Work out the finished part from the listing and answer in its coordinate system (mm). Face numbers are marked on the shaded views. A direction names the side the tool comes from. Give positions to 0.01 mm unless a question says otherwise; leave off trailing zeros. Order: outer loops, then holes, each group sorted by start corner. A loop starts at its lowest first (then second) coordinate and runs counter-clockwise, first axis right, second up. Notation, with made-up numbers: (70.5, 9) - (85.5, 9) arc R9 cw to (85.5, 21) - close; hole circle Ø2 at (41, 2.5). An arc over 180 degrees is marked (long way). Write each question's results on one line, items separated by ' | '.
from build123d import *

# Parameters (mm, degrees)
RESSALTO_EXTRUS_O1_DEPTH  = 15
ESBO_O7_W                 = 30
ESBO_O7_H                 = 15
RESSALTO_EXTRUS_O3_DEPTH  = 3
ESBO_O14_W                = 7
ESBO_O14_H                = 107.753429602
RESSALTO_EXTRUS_O5_DEPTH  = 2
ESBO_O15_W                = 7
ESBO_O15_H                = 107.852923352
RESSALTO_EXTRUS_O6_DEPTH  = 2
ESBO_O16_W                = 7
ESBO_O16_H                = 22.5
RESSALTO_EXTRUS_O9_DEPTH  = 2
CHANFRO11_SIZE            = 20.026147127
CHANFRO11_SIZE_2          = 10
CHANFRO12_SIZE            = 5.181688732
CHANFRO12_SIZE_2          = 10
CHANFRO13_SIZE            = 2
CHANFRO14_SIZE            = 4.8
CHANFRO14_SIZE2           = 5.970145796
CHANFRO16_SIZE            = 1.5
CHANFRO17_SIZE            = 1.5
CHANFRO18_SIZE            = 1
ESBO_O17_R                = 2
CORTE_EXTRUS_O1_DEPTH     = 5
CHANFRO20_SIZE            = 1
RESSALTO_EXTRUS_O10_DEPTH = 7
RESSALTO_EXTRUS_O11_DEPTH = 2
RESSALTO_EXTRUS_O13_DEPTH = 2
ESBO_O23_W                = 5
ESBO_O23_H                = 10
CORTE_EXTRUS_O2_DEPTH     = 60
CHANFRO22_SIZE            = 1.5
CHANFRO21_SIZE            = 1


# Some blends are built 0.0001 mm under size
with BuildPart() as part:
    # Esboço2 → Ressalto-extrusão1 (new body)
    with BuildSketch(Plane.XY):
        Polygon((-41.65, 8.85), (-41.65, 11.85), (-50.65, 11.85), (-50.65, -10.65), (-27.65, -10.65), (-27.65, -7.65), (-47.65, -7.65), (-47.65, 8.85), align=None)
    extrude(amount=RESSALTO_EXTRUS_O1_DEPTH)



with BuildPart() as body_2:
    # Esboço7 → Ressalto-extrusão3 (new body)
    with BuildSketch(Plane(origin=(0, -117.65, 0), x_dir=(-1, 0, 0), z_dir=(0, -1, 0))):
        with Locations((59.65, -7.5)):
            Rectangle(ESBO_O7_W, ESBO_O7_H)
    extrude(amount=-RESSALTO_EXTRUS_O3_DEPTH)


with BuildPart() as part_1:
    add(part.part)

    add(body_2.part)  # Loft3 merges body 2
    # Esboço9 → Loft3 section 0
    with BuildSketch(Plane(origin=(0, -114.65, 0), x_dir=(1, 0, 0), z_dir=(0, 1, 0))):
        with BuildLine():
            Line((-69.65, -15), (-64.65, -15))
            Line((-64.65, -15), (-64.65, 0))
            Line((-64.65, 0), (-69.65, 0))
            Line((-69.65, 0), (-69.65, -15))
        make_face()
    # Esboço8 → Loft3 section 1
    with BuildSketch(Plane.XZ.offset(10.65)):
        with BuildLine():
            Line((-50.65, 15), (-45.65, 15))
            Line((-45.65, 15), (-45.65, 0))
            Line((-45.65, 0), (-50.65, 0))
            Line((-50.65, 0), (-50.65, 15))
        make_face()
    loft()

    # Esboço14 → Ressalto-extrusão5 (add)
    with BuildSketch(Plane(origin=(-42.292744028, 7.726559005, 0), x_dir=(0, 0, -1), z_dir=(0.9837182167305484, -0.17971775113346497, 0))):
        with Locations((-7.5, -70.525331358)):
            Rectangle(ESBO_O14_W, ESBO_O14_H)
    extrude(amount=RESSALTO_EXTRUS_O5_DEPTH)

    # Esboço15 → Ressalto-extrusão6 (add)
    with BuildSketch(Plane(origin=(-47.131251678, 8.610517133, 0), x_dir=(0, 0, 1), z_dir=(-0.9837182167305483, 0.17971775113346522, 0))):
        with Locations((7.5, -73.505764779)):
            Rectangle(ESBO_O15_W, ESBO_O15_H)
    extrude(amount=RESSALTO_EXTRUS_O6_DEPTH)

    # Esboço16 → Ressalto-extrusão9 (add)
    with BuildSketch(Plane.ZY.offset(50.65)):
        with Locations((7.5, 0.6)):
            Rectangle(ESBO_O16_W, ESBO_O16_H)
    extrude(amount=RESSALTO_EXTRUS_O9_DEPTH)

    # Chanfro11
    # the kernel refuses this chamfer: 20.026147127, 10 mm, written as the material it adds along each edge
    with BuildSketch(Plane(origin=(-64.65, -114.65, 55.83646579), x_dir=(0.9998316750706326, -0.018347248443652868, 0), z_dir=(0, 0, -1))) as chanfro11_piece_1_section:
        Polygon((CHANFRO11_SIZE * 0.999831675085, -CHANFRO11_SIZE * 0.0183472484439), (CHANFRO11_SIZE_2 * 0.161638977635, -CHANFRO11_SIZE_2 * 0.986849958661), (0, 0), align=None)
    chanfro11_piece_1 = extrude(amount=55.83646579, mode=Mode.PRIVATE)
    chanfro11_piece_1 = split(chanfro11_piece_1, bisect_by=Plane(origin=(-44.65, -111.70383057, 13), z_dir=(-1, 0, 0)), keep=Keep.TOP, mode=Mode.PRIVATE)
    chanfro11_piece_1 = split(chanfro11_piece_1, bisect_by=Plane(origin=(-56.081001228, -111.70383057, 15), z_dir=(0, 0, -1)), keep=Keep.TOP, mode=Mode.PRIVATE)
    add(chanfro11_piece_1)

    # Chanfro12
    # the kernel refuses this chamfer: 10, 5.181688732 mm, written as the material it adds along each edge
    with BuildSketch(Plane(origin=(-69.65, -114.65, -14.909754714), x_dir=(-0.9981888061534079, -0.06015901653147684, 0), z_dir=(0, 0, 1))) as chanfro12_piece_1_section:
        Polygon((CHANFRO12_SIZE * 0.99818880622, -CHANFRO12_SIZE * 0.0601590165355), (-CHANFRO12_SIZE_2 * 0.238571767911, -CHANFRO12_SIZE_2 * 0.971124869188), (0, 0), align=None)
    chanfro12_piece_1 = extrude(amount=29.909754714, mode=Mode.PRIVATE)
    chanfro12_piece_1 = split(chanfro12_piece_1, bisect_by=Plane(origin=(-74.65, -111.318186465, 5.5), z_dir=(1, 0, 0)), keep=Keep.TOP, mode=Mode.PRIVATE)
    chanfro12_piece_1 = split(chanfro12_piece_1, bisect_by=Plane(origin=(-70.664221075, -111.318186465, 0), z_dir=(0, 0, 1)), keep=Keep.TOP, mode=Mode.PRIVATE)
    add(chanfro12_piece_1)

    # Chanfro13
    chanfro13_edges = [part_1.edges().sort_by_distance(p)[0] for p in [
        (-46.15, 11.85, 15),
        (-46.15, 11.85, 0),
    ]]
    chamfer(chanfro13_edges, length=CHANFRO13_SIZE)

    # Chanfro14
    chanfro14_edges = [part_1.edges().sort_by_distance(p)[0] for p in [
        (-43.616897465, -10.65, 7.5),
    ]]
    chanfro14_side = [part_1.faces().sort_by_distance(p)[0] for p in [
        (-52.309535597, -58.230756092, 7.5),
    ]]
    chamfer(chanfro14_edges, length=CHANFRO14_SIZE, length2=CHANFRO14_SIZE2, reference=chanfro14_side[0])

    # Chanfro16
    chanfro16_edges = [part_1.edges().sort_by_distance(p)[0] for p in [
        (-50.65, 11.85, 3),
        (-51.65, 11.85, 11),
        (-51.65, 11.85, 4),
        (-52.65, 11.85, 7.5),
        (-54.251411244, -57.731408916, 0),
        (-54.251411244, -57.731408916, 15),
        (-53.751411244, -109.724353826, 0),
        (-53.751411244, -109.724353826, 15),
        (-59.251411244, -57.731408916, 15),
        (-59.251411244, -57.731408916, 0),
        (-71.251411244, -109.603357662, 15),
        (-71.251411244, -109.603357662, 0),
        (-50.65, 11.85, 12),
        (-50.65, -0.4, 0),
        (-50.65, 10.85, 1),
        (-50.65, -0.4, 15),
        (-50.65, 10.85, 14),
        (-74.65, -116.021948745, 0),
        (-74.65, -116.021948745, 15),
        (-44.65, -116.14294491, 15),
        (-44.65, -116.14294491, 0),
    ]]
    chamfer(chanfro16_edges, length=CHANFRO16_SIZE)

    # Chanfro17
    chanfro17_edges = [part_1.edges().sort_by_distance(p)[0] for p in [
        (-37.412413451, -10.65, 0),
        (-37.412413451, -10.65, 15),
    ]]
    chamfer(chanfro17_edges, length=CHANFRO17_SIZE)

    # Chanfro18
    chanfro18_edges = [part_1.edges().sort_by_distance(p)[0] for p in [
        (-61.620535422, -59.570685278, 4),
        (-52.65, -0.059403589, 11),
        (-52.7408582, -60.591679812, 4),
        (-61.620535422, -59.570685278, 11),
        (-52.7408582, -60.591679812, 11),
        (-41.06314717, -13.01092372, 4),
        (-41.06314717, -13.01092372, 11),
        (-52.65, -0.059403589, 4),
    ]]
    chamfer(chanfro18_edges, length=CHANFRO18_SIZE)

    # Esboço17 → Corte-extrusão1 (cut)
    with BuildSketch(Plane.XZ.offset(10.65)):
        with Locations(Location((-34.15, 7.5, 0), (0, 0, 270))):
            Circle(ESBO_O17_R)
    extrude(amount=-CORTE_EXTRUS_O1_DEPTH, mode=Mode.SUBTRACT)

    # Chanfro20
    chanfro20_edges = [part_1.edges().sort_by_distance(p)[0] for p in [
        (-41.65, 11.85, 7.5),
        (-41.65, 10.85, 14),
        (-41.65, 10.85, 1),
        (-41.65, 9.35, 15),
        (-27.65, -10.65, 7.5),
        (-27.65, -8.4, 0),
        (-27.65, -8.4, 15),
        (-27.65, -9.9, 14.25),
        (-27.65, -9.9, 0.75),
        (-41.65, 9.35, 0),
    ]]
    chamfer(chanfro20_edges, length=CHANFRO20_SIZE)

    # Esboço18 → Ressalto-extrusão10 (add)
    with BuildSketch(Plane.XY.offset(11)):
        Polygon((-44.65, -114.635889819), (-57.26077437, -102.025115449), (-40.293205201, -9.15), (-44.359410271, -9.15), (-60.698866461, -98.587023358), (-61.558389484, -97.727500335), (-67.574940752, -97.727500335), (-51.65, -10.559403589), (-51.65, 10.35), (-52.65, 10.35), (-52.65, 6.027155141), (-74.65, -114.393897491), (-64.647422179, -114.635889819), align=None)
    extrude(amount=-RESSALTO_EXTRUS_O10_DEPTH)

    # Esboço19 → Ressalto-extrusão11 (add)
    with BuildSketch(Plane(origin=(0, 0, 1.5), x_dir=(-1, 0, 0), z_dir=(0, 0, -1))):
        Polygon((28.65, -10.65), (49.35917828, -22.606449655), (46.90078844, -9.15), (46.90078844, -7.65), (28.65, -7.65), align=None)
    extrude(amount=-RESSALTO_EXTRUS_O11_DEPTH)

    # Esboço21 → Ressalto-extrusão13 (add)
    with BuildSketch(Plane.XY.offset(13.5)):
        Polygon((-28.65, -10.65), (-49.35917828, -22.606449655), (-46.90078844, -9.15), (-46.90078844, -7.65), (-28.65, -7.65), align=None)
    extrude(amount=-RESSALTO_EXTRUS_O13_DEPTH)

    # Esboço23 → Corte-extrusão2 (cut)
    with BuildSketch(Plane(origin=(0, 0, 0), x_dir=(0, 0, -1), z_dir=(1, 0, 0))):
        with Locations((-7.5, -62.65)):
            Rectangle(ESBO_O23_W, ESBO_O23_H)
    extrude(amount=-CORTE_EXTRUS_O2_DEPTH, mode=Mode.SUBTRACT)

    # Chanfro22
    chanfro22_edges = [part_1.edges().sort_by_distance(p)[0] for p in [
        (-55.490352601, -67.65, 10),
        (-54.576891062, -57.65, 10),
        (-54.576891062, -57.65, 5),
        (-55.490352601, -67.65, 5),
    ]]
    chamfer(chanfro22_edges, length=CHANFRO22_SIZE)

    # Chanfro21
    chanfro21_edges = [part_1.edges().sort_by_distance(p)[0] for p in [
        (-50.955387185, -108.330502634, 11),
        (-50.955387185, -108.330502634, 4),
        (-48.997924928, -56.796886925, 11),
        (-48.997924928, -56.796886925, 4),
        (-52.65, 8.18857757, 4),
        (-63.65, -54.183371175, 11),
        (-63.65, -54.183371175, 4),
        (-52.65, 8.18857757, 11),
    ]]
    chamfer(chanfro21_edges, length=CHANFRO21_SIZE - 0.0001)  # a hair under: the kernel refuses the full size

    # Esboço26 → Corte-Revolução1 (revolve, cut)
    with BuildSketch(Plane.XY.offset(7.5), mode=Mode.PRIVATE) as corte_revolu_o1_sk:
        Polygon((-30.65, -11.703246541), (-30.65, -10.65), (-34.15, -7.15), (-34.15, -10.65), (-34.15, -11.703246541), align=None)
    revolve(corte_revolu_o1_sk.sketch.rotate(Axis((-34.15, -7.15, 7.5), (0, -1, 0)), 270), axis=Axis((-34.15, -7.15, 7.5), (0, -1, 0)), mode=Mode.SUBTRACT)


solid = part_1.part
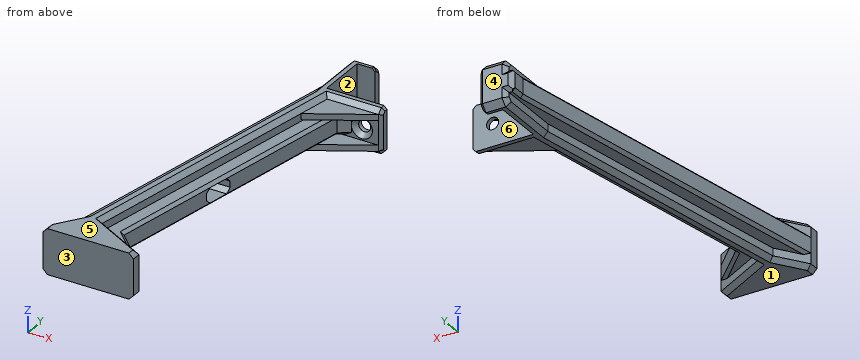
1. A tool of negligible diameter and unlimited length cuts with its end or side. For the marked faces 5 and 6, from which of +Z, -Z, +X, -X, +Y, -Y can it reach the whole face along a straight path? Write none if from no direction.
Answer list:
face 5: +Z, +X, -X, +Y, -Y | face 6: +Z, -Z, +X
2. Given P1, Ø5, axis at x = -34.15, z = 7.5, coming from the -Y side; P2, Ø5.5, axis at x = -38.5, y = -18, coming from the -Z side; P3, Ø2.5, axis at y = -62, z = 8.5, coming from the +X side; P4, Ø5.5, axis at x = -55, y = -62.5, coming from the -Z side, each flat-ended and moving along its own axis, determine where each tip first touches the part or whether it passes through.
Answer list:
P1: y = -9.65 | P2: z = 1.5 | P3: x = -60 | P4: z = 0
3. A cutting plane is placed at A-A, the plane x = -34.15. Write down the section's boundary in (y, z), then the cut area to 3 significant figures.
Answer list:
outline: (-13.83, 1.5) - (-10.65, 1.5) - (-9.15, 0) - (-7.65, 0) - (-7.65, 5.5) - (-9.15, 5.5) - (-10.65, 4) - (-10.65, 3.5) - (-13.83, 3.5) - close; (-13.83, 11.5) - (-10.65, 11.5) - (-10.65, 11) - (-9.15, 9.5) - (-7.65, 9.5) - (-7.65, 15) - (-9.15, 15) - (-10.65, 13.5) - (-13.83, 13.5) - close | area: 41.2 mm^2
4. A cutting plane is placed at B-B, the plane y = -108. Write down the section's boundary in (x, z), then the cut area to 3 significant figures.
Answer list:
outline: (-73.48, 5) - (-72.47, 4) - (-70.11, 4) - (-70.11, 1.5) - (-68.27, 0) - (-60.11, 0) - (-56.95, 1.5) - (-56.95, 4) - (-52.7, 4) - (-51.29, 5) - (-51.29, 10) - (-52.7, 11) - (-56.95, 11) - (-56.95, 13.5) - (-60.11, 15) - (-68.27, 15) - (-70.11, 13.5) - (-70.11, 11) - (-72.47, 11) - (-73.48, 10) - close | area: 251 mm^2
5. Determine the mould class of the marked faces 1, 2, 3 and 4 for opening direction Y: +Y half, -Y half, draft (parallel to the pull), parting line (faces both ways), or undercut.
Answer list:
face 1: draft | face 2: undercut | face 3: -Y half | face 4: +Y half
6. Straight lines are drawn through the part: line 1 (Z direction, x = -55, y = -71.5); line 2 (X direction, y = -8.1, z = 7.5); line 3 (X direction, y = -4, z = 14.75). For each, find the intervals that lie inside material, in ascending order. Write a range as [from, to].
Answer list:
line 1: [4, 11] | line 2: [-55.23, -36.15], [-32.15, -27.65] | line 3: [-49.4, -47.65]
